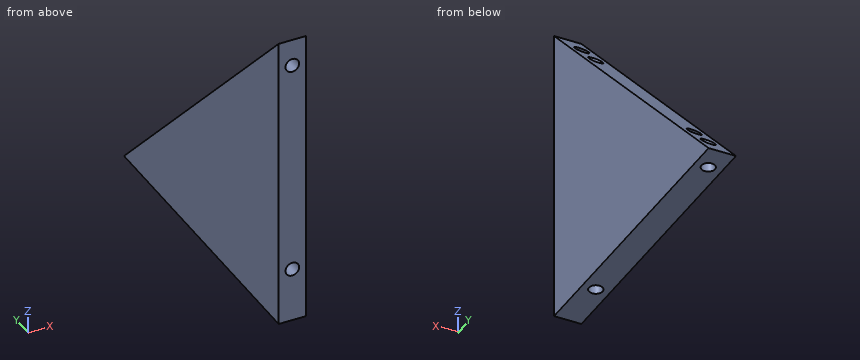
from build123d import *

# Parameters (mm, degrees)
BOSS_EXTRUDE1_DEPTH = 8
SKETCH2_R           = 2
CUT_EXTRUDE1_DEPTH  = 125.707658145
SKETCH3_R           = 2
CUT_EXTRUDE2_DEPTH  = 125.707658145


with BuildPart() as part:
    # Sketch1 → Boss-Extrude1 (new body)
    with BuildSketch(Plane(origin=(0, 0, 0), x_dir=(0, 0, -1), z_dir=(1, 0, 0))):
        Polygon((-88, 0), (0, 0), (0, 88), align=None)
    extrude(amount=BOSS_EXTRUDE1_DEPTH)

    # Sketch2 → Cut-Extrude1 (cut, through all)
    with BuildSketch(Plane(origin=(0, 0, 0), x_dir=(1, 0, 0), z_dir=(0, 1, 0))):
        with Locations(Location((4, -16, 0), (0, 0, 270))):
            Circle(SKETCH2_R)
        with Locations(Location((4, -80, 0), (0, 0, 270))):
            Circle(SKETCH2_R)
    extrude(amount=CUT_EXTRUDE1_DEPTH, mode=Mode.SUBTRACT)

    # Sketch3 → Cut-Extrude2 (cut, through all)
    with BuildSketch(Plane.XY):
        with Locations((4, 16)):
            Circle(SKETCH3_R)
        with Locations(Location((4, 80, 0), (0, 0, 90))):
            Circle(SKETCH3_R)
    extrude(amount=CUT_EXTRUDE2_DEPTH, mode=Mode.SUBTRACT)


solid = part.part
Check sheet for the modelled part. Datum: model origin and axes. Units: mm. Coordinates: 2 decimals unless noted, no trailing zeros. Loops run counter-clockwise (first coordinate to the right, second up) from the corner with the lowest first, then second, coordinate; pieces in that order, holes last. Notation, with made-up numbers: (-7, 13) -> (47, 13) arc R15 cw to (47, 28) -> close; hole circle Ø8 at (6, 15.5). An arc over 180 degrees is marked (long way). Answer in a Markdown table with one row per item.
1. Sectioned sample at B-B, the plane x = 4. Record the boundary of the cut face in (y, z), then the cut area to 3 significant figures.
Check values:
| item | result |
|---|---|
| outline | (0, 0) -> (14, 0) -> (14, 14) -> (0, 14) -> close; (0, 18) -> (14, 18) -> (14, 74) -> (10, 78) -> (0, 78) -> close; (0, 82) -> (6, 82) -> (0, 88) -> close; (18, 0) -> (78, 0) -> (78, 10) -> (74, 14) -> (18, 14) -> close; (18, 18) -> (70, 18) -> (18, 70) -> close; (82, 0) -> (88, 0) -> (82, 6) -> close |
| area | 3,250 mm2 |
2. Material ranges on line 1 along X through (y, z) = (16, 5.75); line 2 along Z through (x, y) = (5, 5); line 3 along Z through (x, y) = (4, 5.5), recorded low to high. Write a range as [from, to].
Check values:
| item | result |
|---|---|
| line 1 | x = [0, 2], [6, 8] |
| line 2 | z = [0, 14.27], [17.73, 78.27], [81.73, 83] |
| line 3 | z = [0, 14], [18, 78], [82, 82.5] |
3. Sectioned sample at A-A, the plane z = 80. Record the boundary of the cut face in (x, y).
Check values:
| item | result |
|---|---|
| outline | (0, 0) -> (2, 0) -> (2, 8) -> (0, 8) -> close; (6, 0) -> (8, 0) -> (8, 8) -> (6, 8) -> close |
4. Sectioned sample at D-D, the plane y = 58. Record the boundary of the cut face in (x, z).
Check values:
| item | result |
|---|---|
| outline | (0, 0) -> (8, 0) -> (8, 30) -> (0, 30) -> close; hole circle Ø4 at (4, 16) |
5. Go/stop test with flat-tipped pins: pin 1 (3.5 mm diameter, centred on x = 4, y = 16, fed in from -Z); pin 2 (3 mm diameter, centred on x = 6.5, y = 76, fed in from +Z). Record where each tip stops, or that it passes through.
Check values:
| item | result |
|---|---|
| pin 1 | passes through |
| pin 2 | stops at z = 13.5 |
6. Sectioned sample at C-C, the plane z = 43. Record the boundary of the cut face in (x, y), then the cut area to 3 significant figures.
Check values:
| item | result |
|---|---|
| outline | (0, 0) -> (8, 0) -> (8, 45) -> (0, 45) -> close; hole circle Ø4 at (4, 16) |
| area | 347 mm2 |
